from build123d import *

# Parameters (mm, degrees)
SKETCH1_W           = 40
SKETCH1_H           = 15
SKETCH1_R           = 4.291657496
BOSS_EXTRUDE1_DEPTH = 2
BOSS_EXTRUDE2_START = -8
SKETCH2_R           = 4.291657496
BOSS_EXTRUDE2_DEPTH = 8


with BuildPart() as part:
    # Sketch1 → Boss-Extrude1 (new body)
    with BuildSketch(Plane(origin=(0, 0, 0), x_dir=(0, 0, -1), z_dir=(1, 0, 0))):
        Rectangle(SKETCH1_W, SKETCH1_H)
        with Locations((-11.747572816, 0)):
            Circle(SKETCH1_R, mode=Mode.SUBTRACT)
        with Locations((11.891261172, -0.124269275)):
            Circle(SKETCH1_R, mode=Mode.SUBTRACT)
    extrude(amount=BOSS_EXTRUDE1_DEPTH)

    # Sketch2 → Boss-Extrude2 (add)
    with BuildSketch(Plane(origin=(2, 0, 0), x_dir=(0, 0, -1), z_dir=(1, 0, 0)).offset(BOSS_EXTRUDE2_START)):
        with Locations((-11.747572816, 0)):
            Circle(SKETCH2_R)
        with Locations((11.891261172, -0.124269275)):
            Circle(SKETCH2_R)
    extrude(amount=BOSS_EXTRUDE2_DEPTH)


solid = part.part
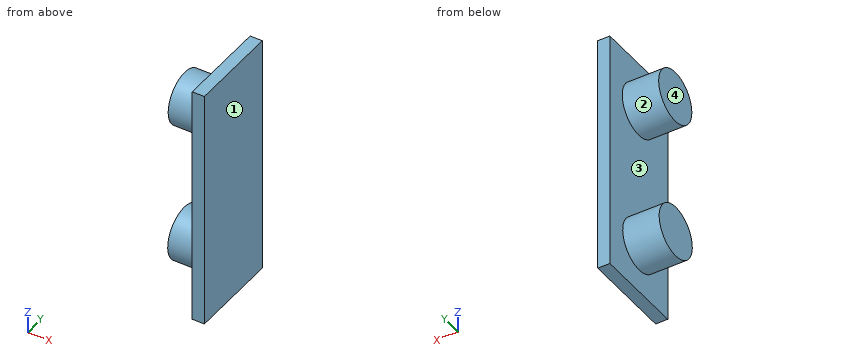
Input: part model. Units: mm. Frame: model coordinates. Face numbers are marked on the shaded views. A direction names the side the tool comes from. Coordinates: 2 decimals unless noted, no trailing zeros. Write each loop counter-clockwise with the first axis right and the second up, starting at its lowest first coordinate (ties: lowest second). Pieces come first, ordered by that corner, then holes. Notation, with made-up numbers: M 45,47.5 L 83,47.5 A25 cw 83,67.5 Z; hole C 83,88 d11. An arc over 180 degrees is marked long. Answer as a JSON object with one key per item and string values. Group by question number.
(1) Section D-D on z = -0.5. Output: boundary loops of the cut face in (x, y).
(2) Section A-A on z = 15. Output: boundary loops of the cut face in (x, y), plus the area to 3 significant figures.
(3) Section B-B on y = 3.25. Output: boundary loops of the cut face in (x, z), plus the area to 3 significant figures.
(4) Contact query for flat-ended pins moving along their axis: P1, Ø4.5, axis at y = 2.5, z = 4, coming from the -X side; P2, Ø4, axis at x = -5, y = 4, coming from the -Z side. Output: stop coordinate, or through.
(5) Section C-C on x = -1.25. Output: boundary loops of the cut face in (y, z).
(6) Ray query, line 1 along X through (y, z) = (-5.25, -5); line 2 along Z through (x, y) = (-3.25, 2.25); line 3 along Z through (x, y) = (-3, -2.75). Return the intervals inside material, ascending. Write a range as [from, to].
(7) Mould query, pull axis Z, two halves, no side actions, for the marked faces 1 and 2. Classes: pulls with the +Z half, pulls with the -Z half, needs draft (parallel to the pull), parting line crosses it, or undercut.
(8) Set-up query: the marked faces 3 and 4. Return all of +Z, -Z, +X, -X, +Y, -Y with unobstructed straight access to the full face (end or side cutting, diameter ignored); none if empty.
Result set:
{
 "1": {"outline": "M 0,-7.5 L 2,-7.5 L 2,7.5 L 0,7.5 Z"},
 "2": {"outline": "M -6,-2.8 L 0,-2.8 L 0,-7.5 L 2,-7.5 L 2,7.5 L 0,7.5 L 0,2.8 L -6,2.8 Z", "area": "63.6 mm2"},
 "3": {"outline": "M -6,-14.54 L 0,-14.54 L 0,-20 L 2,-20 L 2,20 L 0,20 L 0,14.55 L -6,14.55 L -6,8.94 L 0,8.94 L 0,-9.24 L -6,-9.24 Z", "area": "145 mm2"},
 "4": {"P1": "stops at x = 0", "P2": "stops at z = -15.62"},
 "5": {"outline": "C -0.12,-11.89 d8.58; C 0,11.75 d8.58"},
 "6": {"line 1": "x = [0, 2]", "line 2": "z = [-15.47, -8.32], [8.09, 15.4]", "line 3": "z = [-15.29, -8.5], [8.45, 15.04]"},
 "7": {"face 1": "needs draft", "face 2": "undercut"},
 "8": {"face 3": "-X", "face 4": "+Z, -Z, -X, +Y, -Y"}
}
